Read the model definition and answer for the solid it produces. Units are mm, in the model's axes. A direction names the side the tool comes from. Give positions to 0.01 mm unless a question says otherwise; leave off trailing zeros. Order: outer loops, then holes, each group sorted by start corner. A loop starts at its lowest first (then second) coordinate and runs counter-clockwise, first axis right, second up.
```python
from build123d import *

# Parameters (mm, degrees)
F1_DEPTH  = 20
F3_DEPTH  = 4
F5_DEPTH  = 1
F7_DEPTH  = 20.001
F10_W     = 15
F10_H     = 9.1
F11_DEPTH = 1


# Not quite as in the source:
# - a pattern or mirror of a feature is missing from the dataset's text; its kind, count and spacing are read off the source's solid


with BuildPart() as f1:
    # F0 (on Front) → F1 (new body)
    with BuildSketch(Plane.XZ):
        Polygon((-16.45, 3), (-19.25, -1.7), (-18.09, -1.7), (-17.0772340426, 0), (0, 0), (0, 3), align=None)
    extrude(amount=F1_DEPTH)

    # F2 (on face) → F3 (cut)
    with BuildSketch(Plane.XZ.offset(20)):
        Polygon((-16.2, 1), (-0.5, 1), (0, 0.8180148829), (0, 3), (-16, 3), (-16.5, 1.1091910703), align=None)
    f3 = extrude(amount=-F3_DEPTH, mode=Mode.SUBTRACT)

    # F3_copies: F3 across plane
    add(f3.mirror(Plane.ZX.offset(-10)), mode=Mode.SUBTRACT)

    # F4 (on face) → F5 (cut)
    with BuildSketch(Plane.XZ.offset(20)):
        Polygon((0, -1), (0, 0.8180148829), (-0.5, 1), (-16.2, 1), (-16.5, 1.1091910703), (-17.0577483365, -1), align=None)
    f5 = extrude(amount=-F5_DEPTH, mode=Mode.SUBTRACT)

    # F5_copies: F5 across plane
    add(f5.mirror(Plane.ZX.offset(-10)), mode=Mode.SUBTRACT)

    # F6 (on face) → F7 (cut, through all)
    with BuildSketch(Plane.XZ.offset(20)):
        Polygon((-18.67, -1.7), (-18.09, -1.7), (-17.0772340426, 0), (-17.683862779, 0), align=None)
    extrude(amount=-F7_DEPTH, mode=Mode.SUBTRACT)

    # F10 (on face) → F11 (cut)
    with BuildSketch(Plane(origin=(0, 0, 0), x_dir=(1, 0, 0), z_dir=(0, 0, -1))):
        with Locations((-9, 10)):
            Rectangle(F10_W, F10_H)
    extrude(amount=-F11_DEPTH, mode=Mode.SUBTRACT)


solid = f1.part
```
1) The part is cut by section A-A on x = -9.5. Determine the outline of the cut face in (y, z).
Final values:
outline: (-19, 0) - (-14.55, 0) - (-14.55, 1) - (-5.45, 1) - (-5.45, 0) - (-1, 0) - (-1, 1) - (-4, 1) - (-4, 3) - (-16, 3) - (-16, 1) - (-19, 1) - close
2) For a pull along X with two mould halves and no side action, classify faces 4 (the face through (-8, -16, 2)), 5 (the face through (-18.17, -10.14, -0.84)), 6 (the face through (-9, -10, 1)) as released by +X, released by -X, zero draft, split by the parting line, or undercut.
Final values:
face 4: zero draft
face 5: released by +X
face 6: undercut
3) The part is cut by section C-C on z = 1.35. Determine the outline of the cut face in (x, y), and give its area (3 significant figures).
Final values:
outline: (-17.43, -20) - (-16.44, -20) - (-16.44, -16) - (0, -16) - (0, -4) - (-16.44, -4) - (-16.44, 0) - (-17.43, 0) - close
area: 217 mm2
4) Consider L1, parallel to Y at x = -10.25, z = 0.45; L2, parallel to Z at x = -5, y = -3.5; L3, parallel to Z at x = -12, y = -15.25. Determine where each line is inside the solid, lowest interval first.
Final values:
L1: y = -19 to -14.55, -5.45 to -1
L2: z = 0 to 1
L3: z = 0 to 3
5) The part is cut by section D-D on z = 0.3. Determine the outline of the cut face in (x, y).
Final values:
outline: (-18.06, -20) - (-16.71, -20) - (-16.71, -19) - (0, -19) - (0, -1) - (-16.71, -1) - (-16.71, 0) - (-18.06, 0) - close; hole (-16.5, -14.55) - (-1.5, -14.55) - (-1.5, -5.45) - (-16.5, -5.45) - close
6) The part is cut by section B-B on y = -8.75. Determine the outline of the cut face in (x, z), and give its area (3 significant figures).
Final values:
outline: (-19.25, -1.7) - (-18.67, -1.7) - (-17.68, 0) - (-16.5, 0) - (-16.5, 1) - (-1.5, 1) - (-1.5, 0) - (0, 0) - (0, 3) - (-16.45, 3) - close
area: 38.0 mm2
7) A tool of negligible diameter and unlimited length cuts with its end or side. For faces 1 (the face through (-17, 0, 1)), 2 (the face through (-9, -5, 0)), 3 (the face through (-9.1, -5.45, 0.5)), from which of +Z, -Z, +X, -X, +Y, -Y can it reach the whole face along a straight path? Write none if from no direction.
Final values:
face 1: +Z, -Z, +X, -X, +Y
face 2: -Z, +X, +Y, -Y
face 3: -Z
8) Given pin 1 (1.5 mm diameter, centred on y = -10.5, z = 1.5, fed in from -X); pin 2 (8 mm diameter, centred on x = -9, y = -7, fed in from -Z); pin 3 (0.6 mm diameter, centred on x = -11, z = 0.5, fed in from +Y); pin 4 (3.5 mm diameter, centred on x = -8, y = -2.5, fed in from +Z), each flat-ended and moving along its own axis, determine where each tip first touches the part or whether it passes through.
Final values:
pin 1: stops at x = -17.79
pin 2: stops at z = 0
pin 3: stops at y = -1
pin 4: stops at z = 3
